Print and shaded views of the part. All mm, measured from the part's lowest x, y and z. Give positions to 0.01 mm unless a question says otherwise; leave off trailing zeros. Loops run counter-clockwise (first coordinate to the right, second up) from the corner with the lowest first, then second, coordinate; pieces in that order, holes last.
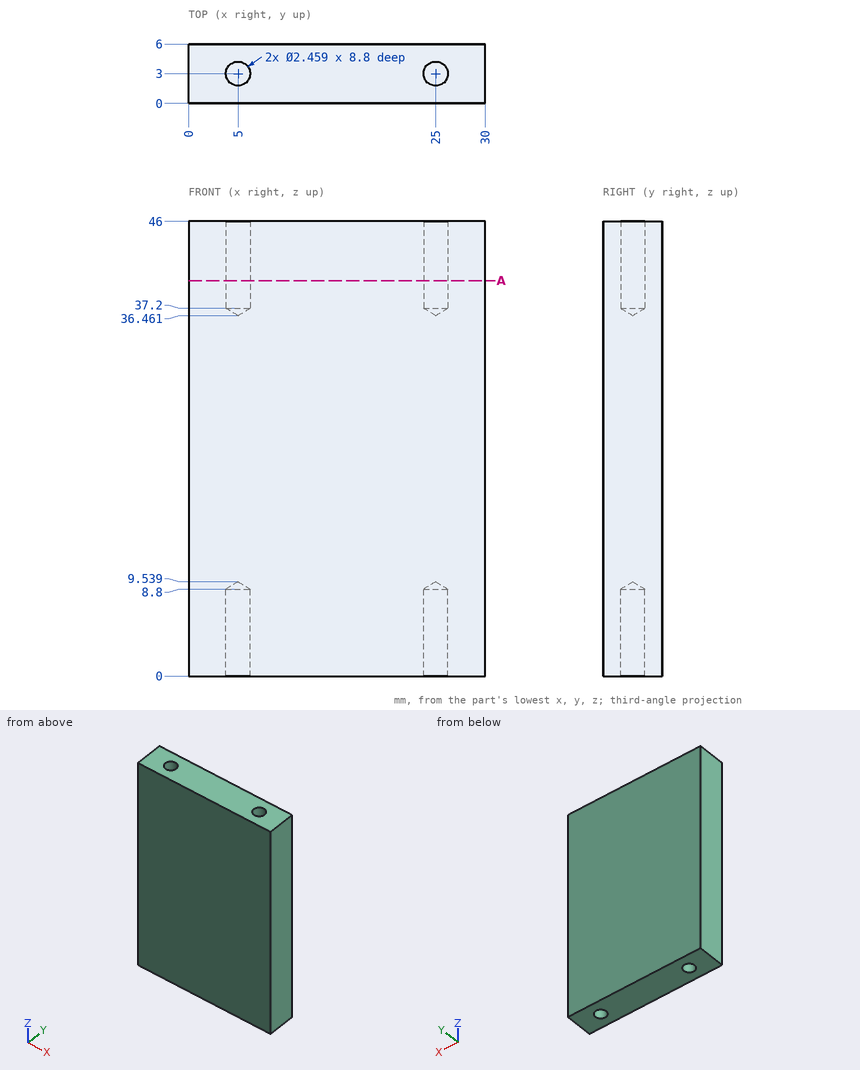
1. Probe line 1 along X through (y, z) = (3, 7); line 2 along X through (y, z) = (2.15, 8); line 3 along Y through (x, z) = (25, 44.25). List the from-to ranges inside material, lowest first.
Responses:
line 1: x = 0 to 3.77, 6.23 to 23.77, 26.23 to 30
line 2: x = 0 to 4.11, 5.89 to 24.11, 25.89 to 30
line 3: y = 0 to 1.77, 4.23 to 6
2. Saw through at A-A, the plane z = 40. List the corners of the cut face in (x, y), and give its area (4 significant figures).
Responses:
outline: (0, 0) - (30, 0) - (30, 6) - (0, 6) - close; hole circle Ø2.46 at (5, 3); hole circle Ø2.46 at (25, 3)
area: 170.5 mm2
3. Drop a flat-ended pin along its axis: pin 1 (2 mm diameter, centred on x = 5, y = 3, fed in from +Z). Give the stop position or say it passes through.
Responses:
pin 1: stops at z = 37.06
